Read the model definition and answer for the solid it produces. Units are mm, in the model's axes. A direction names the side the tool comes from. Give positions to 0.01 mm unless a question says otherwise; leave off trailing zeros. Order: outer loops, then holes, each group sorted by start corner. A loop starts at its lowest first (then second) coordinate and runs counter-clockwise, first axis right, second up. Notation, with made-up numbers: M 79,52.5 L 128,52.5 A14 cw 128,66.5 Z; hole C -24,-27.75 d6. An arc over 180 degrees is marked long. Write item = value, one per line. Start each with the question number.
Autodesk Inventor part; units mm, degrees
ref_plane "YZ Plane" through (0, 0, 0) normal (1, 0, 0) x (0, 1, 0)
ref_plane "XZ Plane" through (0, 0, 0) normal (0, 1, 0) x (-1, 0, 0)
ref_plane "XY Plane" through (0, 0, 0) normal (0, 0, 1) x (1, 0, 0)
sketch "StraightTrack1" plane through (0, 0, 0) normal (0, 0, 1) x (1, 0, 0)
  line L0 (0, 0) -> (304.8, 0)
  line L1 (304.8, 0) -> (304.8, 86.36)
  line L2 (304.8, 86.36) -> (0, 86.36)
  line L3 (0, 86.36) -> (0, 0)
  line L4 (0, 43.18) -> (304.8, 43.18) construction
  line L5 (0, 43.18) -> (-127, 43.18) construction
  line L6 (304.8, 43.18) -> (431.8, 43.18) construction
  line L7 (-35.3212, 50.8) -> (355.1298, 50.8) construction
  line L8 (-9.3356, 35.56) -> (354.8509, 35.56) construction
  circle A0 centre (-25.4, 43.18) radius 17.78
  line L9 (-9.3356, 50.8) -> (0, 50.8)
  line L10 (-9.3356, 35.56) -> (0, 35.56)
  line L11 (-16.6442, 10.16) -> (350.0615, 10.16) construction
  line L12 (-16.6442, 76.2) -> (344.385, 76.2) construction
  line L13 (0, 10.16) -> (304.8, 10.16)
  line L14 (0, 76.2) -> (304.8, 76.2)
  line L15 (0, 67.31) -> (304.8, 67.31)
  line L16 (0, 19.05) -> (304.8, 19.05)
  line L17 (304.8, 50.8) -> (296.8596, 50.8)
  line L18 (304.8, 35.56) -> (296.8596, 35.56)
  circle A1 centre (279.4, 43.18) radius 19.05
  dimension "d0" = 304.8
  dimension "d1" = 86.36
  dimension "d2" = 127
  dimension "d3" = 127
  dimension "d5" = 35.56
  dimension "d6" = 15.24
  dimension "d7" = 35.56
  dimension "d8" = 25.4
  dimension "d9" = 9.3356
  dimension "d10" = 10.16
  dimension "d11" = 10.16
  dimension "d12" = 8.89
  dimension "d13" = 8.89
  dimension "d22" = 38.1
  dimension "d23" = 279.4
extrude "Extrusion1" add sketch "StraightTrack1" against normal blind 25.4 contours L3 L13 L1 L0 | L3 L16 L1 L13 | L3 L15 L1 L17 A1 L18 L16 | L10 A0 L9 L3 | A0 | L3 L14 L1 L15 | L3 L2 L1 L14
extrude "Extrusion3" cut sketch "StraightTrack1" against normal blind 4.7625 contours L3 L16 L1 L13 | L3 L14 L1 L15
fillet "Fillet1" radius 4.826 1 edges at (296.8596, 35.56, -12.7)
fillet "Fillet2" radius 4.826 1 edges at (296.8596, 50.8, -12.7)
fillet "Fillet3" radius 4.826 1 edges at (-9.3356, 50.8, -12.7)
fillet "Fillet4" radius 4.826 1 edges at (-9.3356, 35.56, -12.7)
properties part number "Sun_StraightTrack"
1) Each of these flat-tipped pins is pushed along its axis until it touches: P1, Ø12.5, axis at y = 11, z = -14.5, coming from the -X side; P2, Ø5, axis at x = -4, z = -15, coming from the -Y side; P3, Ø8, axis at x = -4.5, z = -12, coming from the -Y side. Where does it stop, or does it pass through?
2) Find the intervals of material crossed by probe 1 along Y at (x, z) = (72, -4.5); probe 2 along Y at (x, z) = (279.4, -17.75); probe 3 along X at (y, z) = (65, -18), in increasing order. Write a range as [from, to].
3) Find section C-C on z = -21.25. Determine the outline of the cut face in (x, y).
4) For a pull along Y with two mould halves and no side action, classify faces 1 (the face through (0, 69, -13)), 2 (the face through (260.363, 43.871, -12.522)), 3 (the face through (150, 0, -13)) as pulls with the +Y half, pulls with the -Y half, needs draft (parallel to the pull), parting line crosses it, or undercut.
5) Find section A-A on x = 279.4. Determine the outline of the cut face in (y, z).
6) For faces 4 (the face through (128, 44, 0)), 5 (the face through (-3, 35.56, -13)), 6 (the face through (150, 15, -4.762)), 7 (the face through (304.8, 68, -13)), 8 (the face through (-3, 50.8, -13)), determine the directions among +Z, -Z, +X, -X, +Y, -Y from which every point of the face is accessible in a straight line to the end or side of a thin tool.
7) Find section B-B on x = 112.5. Determine the outline of the cut face in (y, z).
8) Find section D-D on y = 81.5. Determine the outline of the cut face in (x, z), plus the area to 3 significant figures.
Numbers:
q1.P1 = 0
q1.P2 = 35.56
q1.P3 = 35.14
q2.probe_1 = [0, 10.16], [19.05, 67.31], [76.2, 86.36]
q2.probe_2 = [0, 24.13], [62.23, 86.36]
q2.probe_3 = [0, 304.8]
q3.outline = M -10.56,33.39 A4.83 cw -6.53,35.56 L 0,35.56 L 0,0 L 304.8,0 L 304.8,35.56 L 299.78,35.56 A4.83 ccw 295.66,33.25 A19.05 cw long 295.66,53.11 A4.83 ccw 299.78,50.8 L 304.8,50.8 L 304.8,86.36 L 0,86.36 L 0,50.8 L -6.53,50.8 A4.83 cw -10.56,52.97 A17.78 ccw long Z
q4.face_1 = needs draft
q4.face_2 = undercut
q4.face_3 = pulls with the -Y half
q5.outline = M 0,-25.4 L 24.13,-25.4 L 24.13,0 L 19.05,0 L 19.05,-4.76 L 10.16,-4.76 L 10.16,0 L 0,0 Z; M 62.23,-25.4 L 86.36,-25.4 L 86.36,0 L 76.2,0 L 76.2,-4.76 L 67.31,-4.76 L 67.31,0 L 62.23,0 Z
q6.face_4 = +Z, +X, -X, +Y, -Y
q6.face_5 = +Z, -Z, -Y
q6.face_6 = +Z, +X, -X
q6.face_7 = +Z, -Z, +X, +Y, -Y
q6.face_8 = +Z, -Z, +Y
q7.outline = M 0,-25.4 L 86.36,-25.4 L 86.36,0 L 76.2,0 L 76.2,-4.76 L 67.31,-4.76 L 67.31,0 L 19.05,0 L 19.05,-4.76 L 10.16,-4.76 L 10.16,0 L 0,0 Z
q8.outline = M 0,-25.4 L 304.8,-25.4 L 304.8,0 L 0,0 Z
q8.area = 7,740 mm2
